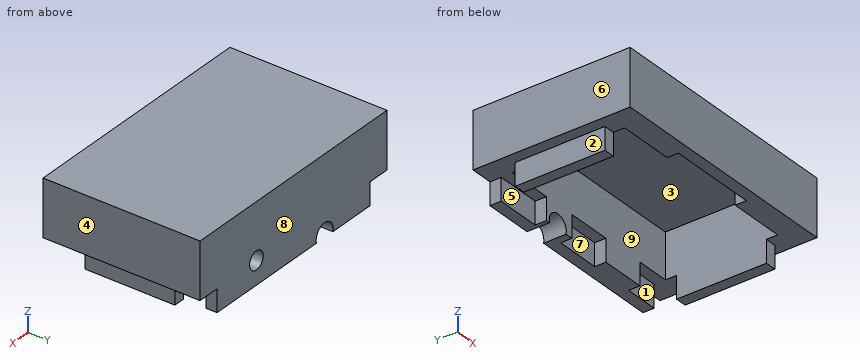
from build123d import *

# Parameters (mm, degrees)
SKETCH1_W           = 110
SKETCH1_H           = 70
BOSS_EXTRUDE1_DEPTH = 5
SKETCH2_W           = 90
SKETCH2_H           = 10
BOSS_EXTRUDE2_DEPTH = 20
SKETCH4_W           = 40
SKETCH4_H           = 10
CUT_EXTRUDE1_DEPTH  = 5
SKETCH5_W           = 5
SKETCH5_H           = 40
BOSS_EXTRUDE4_DEPTH = 10
BOSS_EXTRUDE5_DEPTH = 10
SKETCH7_R           = 5
CUT_EXTRUDE2_DEPTH  = 10
SKETCH8_R           = 4
CUT_EXTRUDE3_DEPTH  = 5


with BuildPart() as part:
    # Sketch1 → Boss-Extrude1 (new body)
    with BuildSketch(Plane.XY):
        with Locations((55, 35)):
            Rectangle(SKETCH1_W, SKETCH1_H)
    extrude(amount=BOSS_EXTRUDE1_DEPTH)

    # Sketch2 → Boss-Extrude2 (add)
    with BuildSketch(Plane(origin=(0, 0, 0), x_dir=(-1, 0, 0), z_dir=(0, 0, -1))):
        with Locations((-55, 65)):
            Rectangle(SKETCH2_W, SKETCH2_H)
        Polygon((-100, 70), (-110, 70), (-110, 0), (-100, 0), (-100, 10), (-100, 60), align=None)
        Polygon((0, 70), (-10, 70), (-10, 60), (-10, 10), (-10, 0), (0, 0), align=None)
        with Locations((-55, 5)):
            Rectangle(SKETCH2_W, SKETCH2_H)
    extrude(amount=BOSS_EXTRUDE2_DEPTH)

    # Sketch4 → Cut-Extrude1 (cut)
    with BuildSketch(Plane(origin=(0, 10, 0), x_dir=(1, 0, 0), z_dir=(0, 1, 0))):
        with Locations((55, 15)):
            Rectangle(SKETCH4_W, SKETCH4_H)
    extrude(amount=-CUT_EXTRUDE1_DEPTH, mode=Mode.SUBTRACT)

    # Sketch5 → Boss-Extrude4 (add)
    with BuildSketch(Plane(origin=(0, 0, -20), x_dir=(-1, 0, 0), z_dir=(0, 0, -1))):
        with Locations((-102.5, 35)):
            Rectangle(SKETCH5_W, SKETCH5_H)
        with Locations((-7.5, 35)):
            Rectangle(SKETCH5_W, SKETCH5_H)
    extrude(amount=BOSS_EXTRUDE4_DEPTH)

    # Sketch6 → Boss-Extrude5 (add)
    with BuildSketch(Plane(origin=(0, 0, -20), x_dir=(-1, 0, 0), z_dir=(0, 0, -1))):
        Polygon((-45, 60), (-30, 60), (-30, 65), (-10, 65), (-10, 70), (-100, 70), (-100, 65), (-85, 65), (-85, 60), (-65, 60), (-65, 65), (-45, 65), align=None)
    extrude(amount=BOSS_EXTRUDE5_DEPTH)

    # Sketch7 → Cut-Extrude2 (cut)
    with BuildSketch(Plane(origin=(0, 70, 0), x_dir=(1, 0, 0), z_dir=(0, 1, 0))):
        with Locations((36.69, 28.79)):
            Circle(SKETCH7_R)
    extrude(amount=-CUT_EXTRUDE2_DEPTH, mode=Mode.SUBTRACT)

    # Sketch8 → Cut-Extrude3 (cut)
    with BuildSketch(Plane(origin=(0, 70, 0), x_dir=(1, 0, 0), z_dir=(0, 1, 0))):
        with Locations(Location((76.88, 19.59, 0), (0, 0, 270))):
            Circle(SKETCH8_R)
    extrude(amount=-CUT_EXTRUDE3_DEPTH, mode=Mode.SUBTRACT)


solid = part.part
Geometry: final body of the model. Coordinates: model frame, mm. Face numbers are marked on the shaded views. A direction names the side the tool comes from. Give positions to 0.01 mm unless a question says otherwise; leave off trailing zeros. Write each loop counter-clockwise with the first axis right and the second up, starting at its lowest first coordinate (ties: lowest second). Pieces come first, ordered by that corner, then holes. Notation, with made-up numbers: (76.25, -5) -> (132.25, -5) arc R23 cw to (132.25, 25) -> close; hole circle Ø10 at (-17.5, 31). An arc over 180 degrees is marked (long way). Answer as a JSON object with one key per item and string values.
1. Contact query for flat-ended pins moving along their axis: pin 1 (4 mm diameter, centred on x = 7, z = -23.5, fed in from -Y); pin 2 (8 mm diameter, centred on x = 18, y = 34.5, fed in from -Z); pin 3 (5.5 mm diameter, centred on y = 62, z = -23.5, fed in from +X). Output: stop coordinate, or through.
Ans:
{"pin 1": "stops at y = 15", "pin 2": "stops at z = 0", "pin 3": "stops at x = 85"}
2. Mould query, pull axis Y, two halves, no side actions, for the marked faces 6, 7, 8 and 9. Classes: pulls with the +Y half, pulls with the -Y half, needs draft (parallel to the pull), parting line crosses it, or undercut.
Ans:
{"face 6": "needs draft", "face 7": "pulls with the -Y half", "face 8": "pulls with the +Y half", "face 9": "undercut"}
3. Cut plane D-D on y = 53.5. Output: boundary loops of the cut face in (x, z), and give its area (3 significant figures).
Ans:
{"outline": "(0, -20) -> (5, -20) -> (5, -30) -> (10, -30) -> (10, 0) -> (100, 0) -> (100, -30) -> (105, -30) -> (105, -20) -> (110, -20) -> (110, 5) -> (0, 5) -> close", "area": "1,050 mm^2"}
4. Cut plane C-C on z = -6. Output: boundary loops of the cut face in (x, y), and give its area (3 significant figures).
Ans:
{"outline": "(0, 0) -> (110, 0) -> (110, 70) -> (0, 70) -> close; hole (10, 10) -> (100, 10) -> (100, 60) -> (10, 60) -> close", "area": "3,200 mm^2"}
5. Cut plane A-A on y = 63. Output: boundary loops of the cut face in (x, z), and give its area (3 significant figures).
Ans:
{"outline": "(0, -20) -> (30, -20) -> (30, -30) -> (31.84, -30) arc R5 cw (long way) to (41.54, -30) -> (45, -30) -> (45, -20) -> (65, -20) -> (65, -30) -> (85, -30) -> (85, -20) -> (110, -20) -> (110, 5) -> (0, 5) -> close", "area": "3,050 mm^2"}
6. Ray query, probe 1 along X at (y, z) = (67.6, -19.59); probe 2 along Y at (x, z) = (85, -16.5); probe 3 along X at (y, z) = (17.5, -27). Return the intervals inside material, ascending. Write a range as from..to.
Ans:
{"probe 1": "x = 0..72.88, 80.88..110", "probe 2": "y = 0..10, 60..70", "probe 3": "x = 5..10, 100..105"}
7. Access query for the marked faces 1, 2, 3, 4 and 5. Directions: +Z, -Z, +X, -X, +Y, -Y. A direction counts if a zero-diameter tool reaches every point of the face in a straight line with its end or side. Return the directions, or none.
Ans:
{"face 1": "-Z, +X, -Y", "face 2": "-Z, -X, +Y, -Y", "face 3": "-Z", "face 4": "+Z, -Z, +X, +Y, -Y", "face 5": "-Z, -X, -Y"}
8. Cut plane B-B on x = 76.88. Output: boundary loops of the cut face in (y, z), and give its area (3 significant figures).
Ans:
{"outline": "(0, -20) -> (10, -20) -> (10, 0) -> (60, 0) -> (60, -30) -> (70, -30) -> (70, -23.59) -> (65, -23.59) -> (65, -15.59) -> (70, -15.59) -> (70, 5) -> (0, 5) -> close", "area": "810 mm^2"}
